Autodesk Inventor part; units mm, degrees
ref_plane "YZ Plane" through (0, 0, 0) normal (1, 0, 0) x (0, 1, 0)
ref_plane "XZ Plane" through (0, 0, 0) normal (0, 1, 0) x (-1, 0, 0)
ref_plane "XY Plane" through (0, 0, 0) normal (0, 0, 1) x (1, 0, 0)
sketch "Sketch_1" plane through (0, 0, 0) normal (0, 0, 1) x (1, 0, 0)
  line L0 (0, 7.5) -> (0, -7.5)
  line L1 (0, -7.5) -> (6.5174, -7.2724)
  arc A0 (6.5174, -7.2724) -> (7, -6.7727) centre (6.5, -6.7727) ccw
  line L2 (7, -6.7727) -> (7, -5.4555)
  arc A1 (7, -5.4555) -> (6.6294, -4.9725) centre (6.5, -5.4555) ccw
  line L3 (6.6294, -4.9725) -> (4, -4.2679)
  line L4 (4, -4.2679) -> (4, 4.2679)
  line L5 (4, 4.2679) -> (6.6294, 4.9725)
  arc A2 (6.6294, 4.9725) -> (7, 5.4555) centre (6.5, 5.4555) ccw
  line L6 (7, 5.4555) -> (7, 6.7727)
  arc A3 (7, 6.7727) -> (6.5174, 7.2724) centre (6.5, 6.7727) ccw
  line L7 (6.5174, 7.2724) -> (0, 7.5)
  point P0 (0, 0)
  point P1 (0, 0)
  dimension "d11" = 4
extrude "Extrusion1" add sketch "Sketch_1" along normal mid plane 10
sketch "Sketch_3" plane through (0, 0, 0) normal (0, 0, 1) x (1, 0, 0)
  line L0 (0, 8.3333) -> (0, 5.141)
  line L1 (0, 5.141) -> (4, 5.3458)
  line L2 (4, 5.3458) -> (4, 0)
  line L3 (4, 0) -> (8, 0)
  line L4 (8, 0) -> (8, 8.3333)
  line L5 (8, 8.3333) -> (0, 8.3333)
  arc A0 (6, 5.4555) -> (6.6294, 4.9725) centre (6.5, 5.4555) ccw
  arc A1 (6.6294, 4.9725) -> (7, 5.4555) centre (6.5, 5.4555) ccw
  line L6 (7, 5.4555) -> (7, 6.7727)
  arc A2 (7, 6.7727) -> (6.5174, 7.2724) centre (6.5, 6.7727) ccw
  arc A3 (6.5174, 7.2724) -> (6, 6.7727) centre (6.5, 6.7727) ccw
  line L7 (6, 6.7727) -> (6, 5.4555)
  line L8 (4, -4.2679) -> (4, 4.2679)
  line L9 (0, 7.5) -> (0, -7.5)
extrude "Extrusion2" cut sketch "Sketch_3" along normal mid plane 6.6667
sketch "Sketch_4" plane through (0, 0, 0) normal (0, 0, 1) x (1, 0, 0)
  line L0 (0, -8.3333) -> (8, -8.3333)
  line L1 (8, -8.3333) -> (8, 0)
  line L2 (8, 0) -> (4, 0)
  line L3 (4, 0) -> (4, -5.3506)
  line L4 (4, -5.3506) -> (0, -5.141)
  line L5 (0, -5.141) -> (0, -8.3333)
  line L6 (6, -5.4555) -> (6, -6.7727)
  arc A0 (6, -6.7727) -> (6.5174, -7.2724) centre (6.5, -6.7727) ccw
  arc A1 (6.5174, -7.2724) -> (7, -6.7727) centre (6.5, -6.7727) ccw
  line L7 (7, -6.7727) -> (7, -5.4555)
  arc A2 (7, -5.4555) -> (6.6294, -4.9725) centre (6.5, -5.4555) ccw
  arc A3 (6.6294, -4.9725) -> (6, -5.4555) centre (6.5, -5.4555) ccw
  line L8 (4, -4.2679) -> (4, 4.2679)
  line L9 (0, 7.5) -> (0, -7.5)
extrude "Extrusion3" cut sketch "Sketch_4" along normal mid plane 6.6667
sketch "Sketch_5" plane through (0, 0, 0) normal (0, 0, 1) x (1, 0, 0)
  line L0 (4, 0) -> (0, 0)
  line L1 (0, 0) -> (0, 2)
  line L2 (0, 2) -> (1.5, 2)
  line L3 (1.5, 2) -> (1.5, 3.6)
  line L4 (1.5, 3.6) -> (4, 3.6)
  line L5 (4, 3.6) -> (4, 0)
  line L6 (4, 0) -> (0, 0)
  line L7 (7, 5.4555) -> (7, 6.7727)
  line L8 (4, -4.2679) -> (4, 4.2679)
  line L9 (0, 7.5) -> (0, -7.5)
  dimension "d7" = 2
  dimension "d8" = 3.6
  dimension "d9" = 5.5
revolve "Revolution1" cut sketch "Sketch_5" angle 360 about axis through (4, 0, 0) along (1, 0, 0)
properties part number "520022598" material "PA 6.6-MO*Nylatron GS"
Geometry: final body of the model. Coordinates: model frame, mm. A direction names the side the tool comes from. Round coordinates to 2 decimals unless told otherwise and drop trailing zeros. Loops run counter-clockwise (first coordinate to the right, second up) from the corner with the lowest first, then second, coordinate; pieces in that order, holes last. Notation, with made-up numbers: (22.25, -31.75) -> (76.25, -31.75) arc R12 ccw to (76.25, -16.75) -> close; hole circle Ø9 at (70, -24.75). An arc over 180 degrees is marked (long way). Use one line per item in the form item = value. Start each with the question number.
1) First-contact query: P1, Ø1.1, axis at y = 6, z = -0.5, coming from the -X side; P2, Ø5, axis at y = 1, z = 1.5, coming from the -X side; P3, Ø3, axis at y = 1.5, z = 1, coming from the +X side. Flat tips, straight axial feed; report the tip coordinate or a pass-through.
2) Draft query along Y for faces 5 (the flat face through (3, 0, 5)), 6 (the flat face through (1.5, 2, -2)), 7 (the flat face through (1.97, 5.24, -0.05)). Return one class per face: released by +Y, released by -Y, zero draft, split by the parting line, or undercut.
3) Section A-A on z = 0. Output: boundary loops of the cut face in (x, y), then the cut area to 3 significant figures.
4) Section D-D on y = 6.5. Output: boundary loops of the cut face in (x, z).
5) Section B-B on y = 0. Output: boundary loops of the cut face in (x, z), then the cut area to 3 significant figures.
6) Line query: L1, parallel to Z at x = 1.1, y = 0; L2, parallel to Z at x = 2.1, y = 0; L3, parallel to X at y = 5.5, z = -3.25. Output: solid intervals per line, ascending.
7) Access query for faces 1 (the cylindrical face through (1, 0, -2)), 2 (the cylindrical face through (2.768, 3.434, 1.081)), 3 (the flat face through (5.296, 4.615, -4.178)), 4 (the flat face through (6, -6, 0)). Directions: +Z, -Z, +X, -X, +Y, -Y. A direction counts if a zero-diameter tool reaches every point of the face in a straight line with its end or side. Return the directions, or none.
8) Section C-C on x = 1.75. Output: boundary loops of the cut face in (y, z).
Response:
q1.P1 = 6
q1.P2 = 0
q1.P3 = 1.5
q2.face_5 = zero draft
q2.face_6 = undercut
q2.face_7 = released by +Y
q3.outline = (0, -5.14) -> (4, -5.35) -> (4, -3.6) -> (1.5, -3.6) -> (1.5, -2) -> (0, -2) -> close; (0, 2) -> (1.5, 2) -> (1.5, 3.6) -> (4, 3.6) -> (4, 5.35) -> (0, 5.14) -> close; (6, -6.77) arc R0.5 ccw to (6.52, -7.27) arc R0.5 ccw to (7, -6.77) -> (7, -5.46) arc R0.5 ccw to (6.63, -4.97) arc R0.5 ccw to (6, -5.46) -> close; (6, 5.46) arc R0.5 ccw to (6.63, 4.97) arc R0.5 ccw to (7, 5.46) -> (7, 6.77) arc R0.5 ccw to (6.52, 7.27) arc R0.5 ccw to (6, 6.77) -> close
q3.area = 22.2 mm^2
q4.outline = (0, -5) -> (7, -5) -> (7, 5) -> (0, 5) -> (0, 3.33) -> (6, 3.33) -> (6, -3.33) -> (0, -3.33) -> close
q5.outline = (0, -5) -> (4, -5) -> (4, -3.6) -> (1.5, -3.6) -> (1.5, -2) -> (0, -2) -> close; (0, 2) -> (1.5, 2) -> (1.5, 3.6) -> (4, 3.6) -> (4, 5) -> (0, 5) -> close
q5.area = 16.0 mm^2
q6.L1 = -5 to -2, 2 to 5
q6.L2 = -5 to -3.6, 3.6 to 5
q6.L3 = 6 to 7
q7.face_1 = +X, -X
q7.face_2 = +X
q7.face_3 = +Z, -Z, +X
q7.face_4 = -X, +Y, -Y
q8.outline = (-7.44, -5) -> (7.44, -5) -> (7.44, -3.33) -> (5.23, -3.33) -> (5.23, 3.33) -> (7.44, 3.33) -> (7.44, 5) -> (-7.44, 5) -> (-7.44, 3.33) -> (-5.23, 3.33) -> (-5.23, -3.33) -> (-7.44, -3.33) -> close; hole circle Ø7.2 at (0, 0)
